Here's how the part is built. I have some questions about the finished solid (model axes, mm). A direction names the side the tool comes from. Coordinates: 2 decimals unless noted, no trailing zeros. Order: outer loops, then holes, each group sorted by start corner. A loop starts at its lowest first (then second) coordinate and runs counter-clockwise, first axis right, second up. Notation, with made-up numbers: (24.5, -7) - (46.5, -7) arc R21 cw to (46.5, 7) - close; hole circle Ø8 at (-40, 0.25). An arc over 180 degrees is marked (long way). Answer in a Markdown table with one row per item. Add a question column.
Item 1: I want a section at C-C (y = -8). Please give me the cut outline in (x, z).
Item 2: Thinking about a two-plate mould opening in X: for faces 4 (the flat face through (-19, 6, -10)), 5 (the cylindrical face through (24, -23, -10)), 6 (the cylindrical face through (4, 5, -10)), which applies, +X half, -X half, draft (parallel to the pull), parting line (faces both ways), or undercut?
Item 3: On a 3-axis mill with a long thin cutter (end or side, diameter ignored), from which of +Z, -Z, +X, -X, +Y, -Y can I reach the whole of each face in a straight line? I mean faces 1 (the cylindrical face through (31.14, -4.9, -9.86)), 2 (the cylindrical face through (8, -23, -10)), 3 (the cylindrical face through (-0.5, -1.1, -9.9)). Say none if no direction works.
Item 4: Will these pins go through, and if not, where does the flat tip stop? pin 1 Ø6 at (y, z) = (-18, -12) entering from -X; pin 2 Ø9.5 at (x, z) = (-5.5, -10) entering from +Y; pin 3 Ø1 at (x, z) = (13.5, -11.5) entering from +Y; pin 4 Ø4 at (x, y) = (-17.5, -3) entering from +Z.
Item 5: If I drill on line 1 along X through (y, z) = (-15.5, -7.25); line 2 along Z through (x, y) = (-5.5, 4.3); line 3 along Y through (x, z) = (-35, -10), over which ranges is the centre line in solid material (lowest first)? Write a range as from..to.
Item 6: I want a section at B-B (z = -10). Count the separate pieces of the cut face and the enclosed holes in it, plus the area to 3 significant figures.
Item 7: I want a section at A-A (x = -25.5). Please give me the cut outline in (y, z).
Autodesk Inventor part; units mm, degrees
ref_plane "YZ Plane" through (0, 0, 0) normal (1, 0, 0) x (0, 1, 0)
ref_plane "XZ Plane" through (0, 0, 0) normal (0, 1, 0) x (-1, 0, 0)
ref_plane "XY Plane" through (0, 0, 0) normal (0, 0, 1) x (1, 0, 0)
sketch "Sketch1" plane through (0, 0, 0) normal (0, 1, 0) x (-1, 0, 0)
  line L0 (0, 0) -> (40, 0)
  line L1 (40, 0) -> (40, -20)
  line L2 (40, -20) -> (0, -20)
  line L3 (0, -20) -> (0, 0)
  dimension "d0" = 40
  dimension "d1" = 20
extrude "Extrusion1" add sketch "Sketch1" along normal blind 6
sketch "Sketch2" plane through (0, 6, 0) normal (0, 1, 0) x (1, 0, 0)
  line L0 (0, 0) -> (6, 0)
  line L1 (6, 0) -> (6, 20)
  line L2 (6, 20) -> (0, 20)
  line L3 (0, 20) -> (0, 0)
  dimension "d4" = 6
  dimension "d5" = 20
extrude "Extrusion2" add sketch "Sketch2" against normal blind 30
fillet "Fillet1" radius 5 1 edges at (0, 0, -10)
fillet "Fillet4" radius 5 1 edges at (6, 6, -10)
sketch "Sketch5" plane through (0, 0, 0) normal (0, -1, 0) x (1, 0, 0)
  circle A0 centre (-5.5, -10) radius 3
  line L0 (-40, -20) -> (-40, 0)
  line L1 (-5, -20) -> (-40, -20)
  line L2 (6, -20) -> (6, 0)
  circle A1 centre (-25.5, -10) radius 3
  line L3 (-40, 0) -> (-5, 0)
  point P0 (0, 0)
  dimension "d18" = 6
  dimension "d20" = 10
  dimension "d47" = 11.5
  dimension "d48" = 6
  dimension "d49" = 20
  dimension "d50" = 10
fillet "Fillet7" radius 2 2 edges at (-40, 3, 0) (-40, 3, -20)
sketch "Sketch8" plane through (0, -24, -20) normal (-1, 0, 0) x (0, 0, 1)
  line L0 (20, 0) -> (0, 0)
  line L1 (0, 0) -> (20, 0)
  line L2 (20, 0) -> (20, -6)
  line L3 (20, -6) -> (0, -6)
  line L4 (0, -6) -> (0, 0)
  point P0 (20, 24)
  dimension "d35" = 6
extrude "Extrusion6" add sketch "Sketch8" against normal blind 32
fillet "Fillet8" radius 5 1 edges at (0, -30, -10)
fillet "Fillet9" radius 5 1 edges at (6, -24, -10)
sketch "Sketch9" plane through (32, -24, 0) normal (0, 1, 0) x (1, 0, 0)
  line L0 (0, 20) -> (0, 0)
  line L1 (0, 20) -> (-6, 20)
  line L2 (-6, 20) -> (-6, 0)
  line L3 (-6, 0) -> (0, 0)
  line L4 (0, 0) -> (0, 20)
  point P0 (-32, 0)
  dimension "d40" = 6
  dimension "d41" = 20
extrude "Extrusion7" add sketch "Sketch9" along normal blind 20
fillet "Fillet10" radius 5 1 edges at (26, -24, -10)
fillet "Fillet11" radius 5 1 edges at (32, -30, -10)
fillet "Fillet12" radius 3 2 edges at (26, -4, -10) (32, -4, -10)
extrude "Extrusion8" cut sketch "Sketch5" against normal through all both and the other way through all
sketch "Sketch10" plane through (0, 0, 0) normal (0, -1, 0) x (1, 0, 0)
  circle A0 centre (-5.5, -10) radius 3
  circle A1 centre (-5.5, -10) radius 5
  point P0 (0, 0)
  dimension "d53" = 10
extrude "Extrusion9" cut sketch "Sketch10" along normal through all contours A0 | A1
properties part number "Cable_Guide_Holder"
Values follow:
| question | item | result |
|---|---|---|
| 1 | outline | (0, -20) - (6, -20) - (6, 0) - (0, 0) - close; (26, -20) - (32, -20) - (32, 0) - (26, 0) - close |
| 2 | face 4 | draft |
| 2 | face 5 | undercut |
| 2 | face 6 | +X half |
| 3 | face 1 | +Z, -Z, +X, +Y |
| 3 | face 2 | +Z, -Z, +Y |
| 3 | face 3 | -X, -Y |
| 4 | pin 1 | stops at x = 0 |
| 4 | pin 2 | stops at y = 6 |
| 4 | pin 3 | stops at y = -24 |
| 4 | pin 4 | passes through |
| 5 | line 1 | x = 0..6, 26..32 |
| 5 | line 2 | z = -20..-13, -7..0 |
| 5 | line 3 | y = 0..6 |
| 6 | separate pieces | 3 |
| 6 | enclosed holes | 0 |
| 6 | area | 653 mm^2 |
| 7 | outline | (0, -20) - (6, -20) - (6, -13) - (0, -13) - close; (0, -7) - (6, -7) - (6, 0) - (0, 0) - close |
